Geometry check sheet. Reference: the model listing, model coordinates, mm. Face numbers are marked on the shaded views. A direction names the side the tool comes from. Round coordinates to 2 decimals unless told otherwise and drop trailing zeros. Loops run counter-clockwise (first coordinate to the right, second up) from the corner with the lowest first, then second, coordinate; pieces in that order, holes last. Notation, with made-up numbers: (30.25, 44) - (84.25, 44) arc R19 cw to (84.25, 61) - close; hole circle Ø6 at (-10.5, -16). An arc over 180 degrees is marked (long way). Write item = value, one per line.
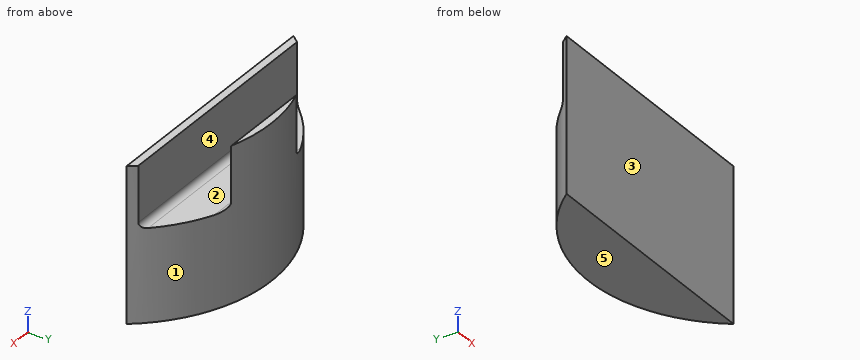
```python
from build123d import *

# Parameters (mm, degrees)
F1_DEPTH = 63.5
F2_W     = 19.05
F2_H     = 25.4
F3_DEPTH = 50.8
F4_R     = 2.54


with BuildPart() as f1:
    # F0 (on Top) → F1 (new body)
    with BuildSketch(Plane.XY):
        with BuildLine():
            Line((-50.8, 0), (50.8, 0))
            ThreePointArc((50.8, 0), (0, 25.4), (-50.8, 0))
        make_face()
    extrude(amount=F1_DEPTH)

    # F2 (on Right) → F3 (cut, symmetric)
    with BuildSketch(Plane.YZ):
        with Locations((12.7, 50.8)):
            Rectangle(F2_W, F2_H)
    extrude(amount=F3_DEPTH, both=True, mode=Mode.SUBTRACT)

    # F4
    f4_edges = [f1.edges().sort_by_distance(p)[0] for p in [
        (0, 3.175, 38.1),
        (0, 22.225, 38.1),
    ]]
    fillet(f4_edges, radius=F4_R)


solid = f1.part
```
(1) Section check A-A (z = 52.5). Enter the section's corners in (x, y) (3 decimals), then the cut area to 3 significant figures.
Answers follow:
outline = (-50.8, 0) - (50.8, 0) arc R63.5 ccw to (48.256, 3.175) - (-48.256, 3.175) arc R63.5 ccw to start; (-19.828, 22.225) - (19.828, 22.225) arc R63.5 ccw to start
area = 399 mm²
(2) Section check D-D (z = 13.5). Enter the section's corners in (x, y).
Answers follow:
outline = (-50.8, 0) - (50.8, 0) arc R63.5 ccw to start
(3) Section check B-B (x = -27.5). Enter the section's corners in (y, z) (3 decimals).
Answers follow:
outline = (0, 0) - (19.136, 0) - (19.136, 38.1) - (5.715, 38.1) arc R2.54 cw to (3.175, 40.64) - (3.175, 63.5) - (0, 63.5) - close
(4) Scan lines: L1, parallel to Y at x = -1.5, z = 6.5; L2, parallel to Z at x = -7.5, y = 18.25; L3, parallel to Y at x = 44.5, z = 46 (3 decimals). Record each from-to range of solid material in increasing order. Write a range as [from, to].
Answers follow:
L1 = [0, 25.38]
L2 = [0, 38.1]
L3 = [0, 3.175]
(5) Mould release check, pull along Y, two halves, no side actions. Record for the marked faces 3, 4 and 5: pulls with the +Y half, pulls with the -Y half, needs draft (parallel to the pull), parting line crosses it, or undercut.
Answers follow:
face_3 = pulls with the -Y half
face_4 = undercut
face_5 = needs draft
(6) Gauge pin test, flat ends, axial feed: pin 1 (3 mm diameter, centred on y = 4.5, z = 51.5, fed in from +X); pin 2 (12 mm diameter, centred on x = -26.5, z = 12.5, fed in from +Y); pin 3 (5 mm diameter, centred on y = 11, z = 8, fed in from +X). Record the tip position at first contact, or that the pin passes through.
Answers follow:
pin_1 = 48.4
pin_2 = 22
pin_3 = 43.14
(7) Section check C-C (y = 16.5). Enter the section's corners in (x, z), then the cut area to 3 significant figures.
Answers follow:
outline = (-32.42, 0) - (32.42, 0) - (32.42, 38.1) - (-32.42, 38.1) - close
area = 2,470 mm²
(8) Set-up check for the marked faces 1 and 2: record each of +Z, -Z, +X, -X, +Y, -Y from which the full face is reachable in a straight line by a thin tool's end or side.
Answers follow:
face_1 = +Z, -Z, +Y
face_2 = +Z, +X, -X
